Geometry check sheet. Reference: drawing and pictorial views, mm from the part's lowest x, y, z. A direction names the side the tool comes from. Give positions to 0.01 mm unless a question says otherwise; leave off trailing zeros. Order: outer loops, then holes, each group sorted by start corner. A loop starts at its lowest first (then second) coordinate and runs counter-clockwise, first axis right, second up.
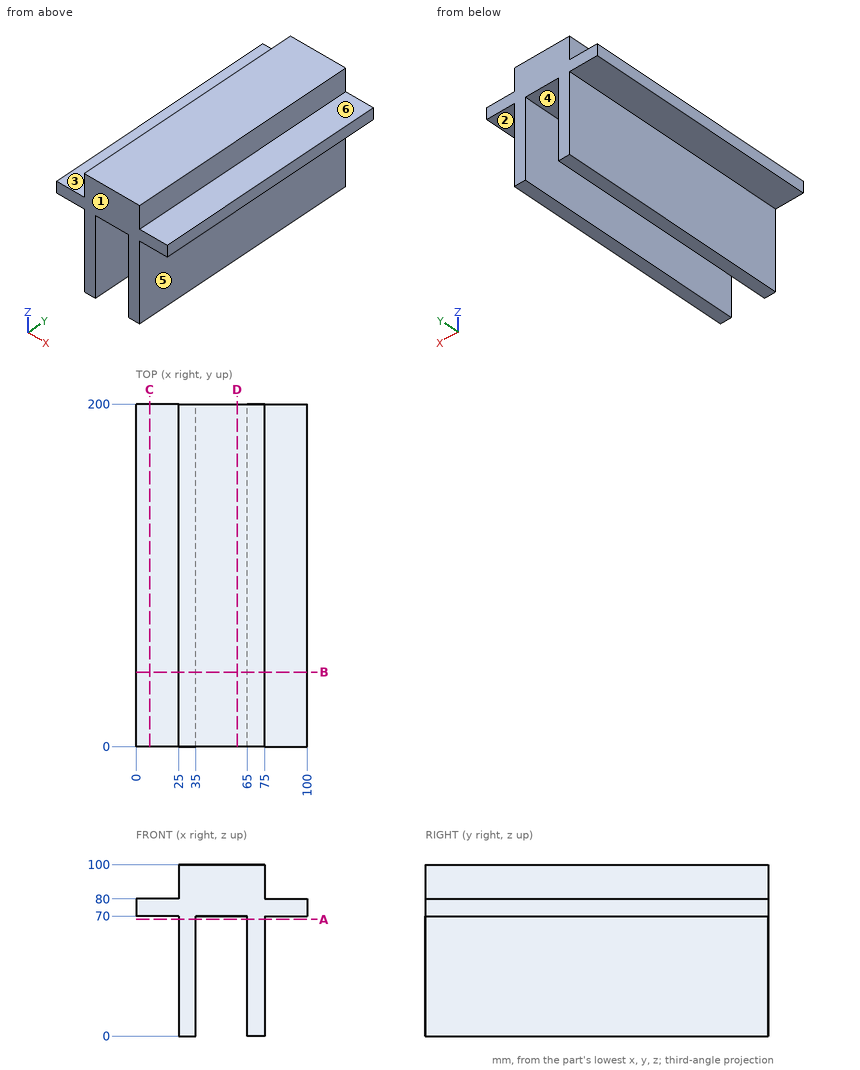
(1) Cross-section at D-D on x = 59. Enter the section's corners in (y, z).
Response values:
outline: (0, 70) - (200, 70) - (200, 100) - (0, 100) - close
(2) Cross-section at A-A on z = 68. Enter the section's corners in (x, y), then the cut area to 3 significant figures.
Response values:
outline: (25, 0) - (35, 0) - (35, 200) - (25, 200) - close; (65, 0) - (75, 0) - (75, 200) - (65, 200) - close
area: 4,000 mm2
(3) Set-up check for the marked faces 4, 5 and 6: record each of +Z, -Z, +X, -X, +Y, -Y from which the full face is reachable in a straight line by a thin tool's end or side.
Response values:
face 4: -Z, +Y, -Y
face 5: -Z, +X, +Y, -Y
face 6: +Z, +X, +Y, -Y
(4) Material ranges on L1, parallel to X at y = 110, z = 46; L2, parallel to Z at x = 90.5, y = 96; L3, parallel to X at y = 154, z = 83, recorded low to high.
Response values:
L1: x = 25 to 35, 65 to 75
L2: z = 70 to 80
L3: x = 25 to 75
(5) Cross-section at B-B on y = 43.5. Enter the section's corners in (x, z).
Response values:
outline: (0, 70) - (25, 70) - (25, 0) - (35, 0) - (35, 70) - (65, 70) - (65, 0) - (75, 0) - (75, 70) - (100, 70) - (100, 80) - (75, 80) - (75, 100) - (25, 100) - (25, 80) - (0, 80) - close
(6) Release check for a two-part mould opening along Z. For the marked faces 1, 2 and 3 record: released by +Z, released by -Z, zero draft, split by the parting line, or undercut.
Response values:
face 1: zero draft
face 2: released by -Z
face 3: released by +Z
(7) Cross-section at C-C on x = 8. Enter the section's corners in (y, z).
Response values:
outline: (0, 70) - (200, 70) - (200, 80) - (0, 80) - close
(8) Gauge pin test, flat ends, axial feed: pin 1 Ø20 at (x, y) = (86.5, 92.5) entering from +Z; pin 2 Ø24 at (x, y) = (46.5, 115) entering from -Z; pin 3 Ø6 at (y, z) = (101, 94.5) entering from -X; pin 4 Ø21 at (y, z) = (123, 31) entering from +X. Record the tip position at first contact, or that the pin passes through.
Response values:
pin 1: stops at z = 80
pin 2: stops at z = 0
pin 3: stops at x = 25
pin 4: stops at x = 75
